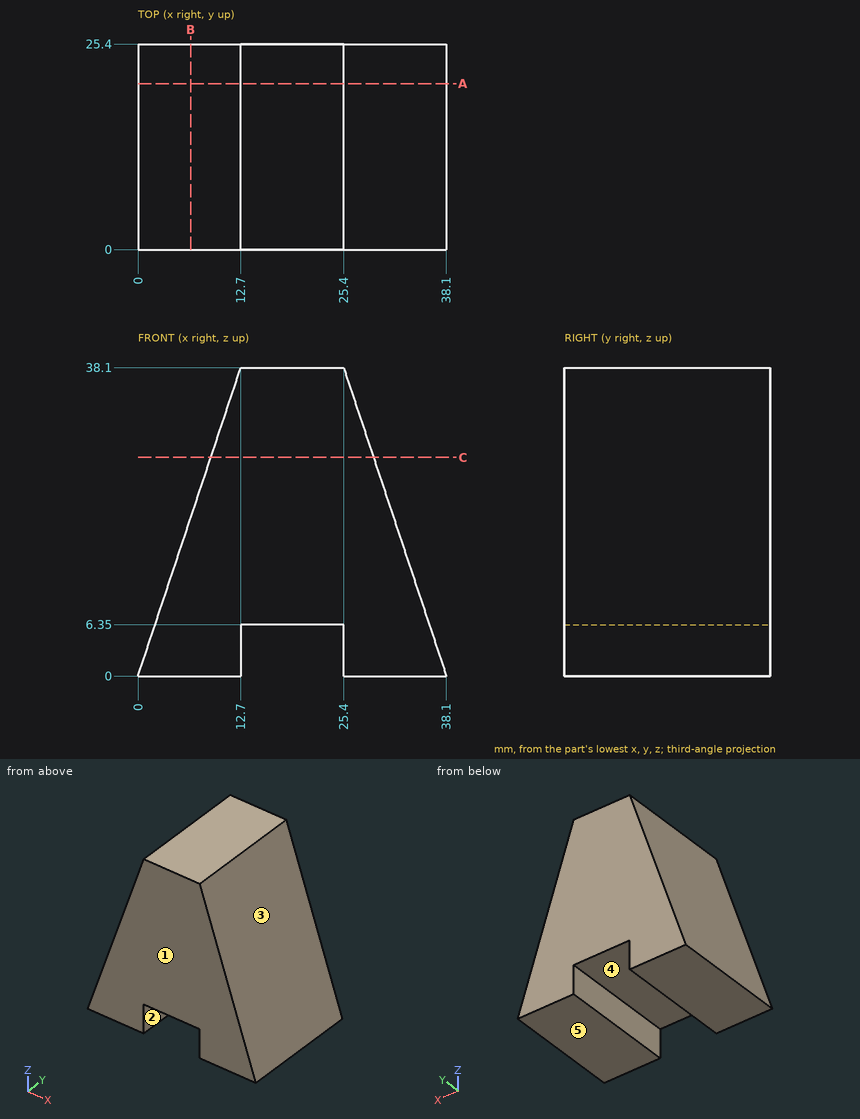
The drawing under review shows one solid part. Ordinate dimensions are in mm from its lowest x, y, z. A direction names the side the tool comes from. Round coordinates to 2 decimals unless told otherwise and drop trailing zeros. Order: outer loops, then holes, each group sorted by start corner. A loop starts at its lowest first (then second) coordinate and runs counter-clockwise, first axis right, second up. Notation, with made-up numbers: (82, 49.5) -> (109, 49.5) arc R32 ccw to (109, 77.5) -> close; hole circle Ø8 at (-25.75, 30). An arc over 180 degrees is marked (long way). Return JSON: item names as keys, results as strings.
1. Insertion check: P1, Ø8, axis at y = 17, z = 8, coming from the +X side; P2, Ø1, axis at x = 34.5, z = 16.5, coming from the +Y side; P3, Ø7, axis at y = 8.5, z = 4.5, coming from the +X side; P4, Ø1.5, axis at y = 16, z = 28, coming from the +X side. Each pin has a flat end and moves straight along its axis. Give the tip position at first contact, or say it passes through.
Answer block:
{"P1": "stops at x = 36.77", "P2": "passes through", "P3": "stops at x = 37.77", "P4": "stops at x = 29.02"}
2. The part is to be moulded in two halves that separate along X. For the marked faces 1, 2 and 3, say which applies: +X half, -X half, draft (parallel to the pull), parting line (faces both ways), or undercut.
Answer block:
{"face 1": "draft", "face 2": "undercut", "face 3": "+X half"}
3. For the marked faces 4 and 5, list the 3-axis set-ups (+Z, -Z, +X, -X, +Y, -Y) from which the entire face can be reached by the end or side of a thin tool; tool diameter is ignored.
Answer block:
{"face 4": "-Z, +Y, -Y", "face 5": "-Z, +X, -X, +Y, -Y"}
4. Take a section at C-C (z = 27). Write out the cut boundary in (x, y), then the cut area to 3 significant figures.
Answer block:
{"outline": "(9, 0) -> (29.1, 0) -> (29.1, 25.4) -> (9, 25.4) -> close", "area": "511 mm²"}
5. Take a section at A-A (y = 20.5). Write out the cut boundary in (x, z).
Answer block:
{"outline": "(0, 0) -> (12.7, 0) -> (12.7, 6.35) -> (25.4, 6.35) -> (25.4, 0) -> (38.1, 0) -> (25.4, 38.1) -> (12.7, 38.1) -> close"}
6. For L1, parallel to Z at x = 21.5, y = 3; L2, parallel to X at y = 16.5, z = 32; L3, parallel to X at y = 4.5, z = 32.5, list the stretches that pass through material, from the lowest coordinate up. Write a range as [from, to].
Answer block:
{"L1": "z = [6.35, 38.1]", "L2": "x = [10.67, 27.43]", "L3": "x = [10.83, 27.27]"}
7. Take a section at B-B (x = 6.5). Write out the cut boundary in (y, z), then the cut area to 3 significant figures.
Answer block:
{"outline": "(0, 0) -> (25.4, 0) -> (25.4, 19.5) -> (0, 19.5) -> close", "area": "495 mm²"}
